Here's how the part is built. I have some questions about the finished solid (model axes, mm). Round coordinates to 2 decimals unless told otherwise and drop trailing zeros. Write each loop counter-clockwise with the first axis right and the second up, starting at its lowest first coordinate (ties: lowest second). Pieces come first, ordered by that corner, then holes. Notation, with made-up numbers: (66.25, 63) -> (117.25, 63) arc R26 cw to (117.25, 93) -> close; hole circle Ø10 at (74, -21). An arc over 180 degrees is marked (long way). Put each result on its own line as item: value. Start each with the question number.
1) If I drill on line 1 along Y through (x, z) = (30, 0.35); line 2 along Y through (x, z) = (50, 2); line 3 along Y through (x, z) = (-10, 0.05), over which ranges is the centre line in solid material (lowest first)? Write a range as [from, to].
2) I want a section at D-D, the plane x = 50. List the corners of the cut face in (y, z) for me.
3) I want a section at B-B, the plane x = 90. List the corners of the cut face in (y, z) for me, then the cut area to 3 significant figures.
4) Will this pin go through, and if not, where does the flat tip stop? P1, Ø5.5, axis at x = 90, y = -52.5, coming from the -Z side.
5) I want a section at A-A, the plane z = 0. List the corners of the cut face in (x, y) for me, then the cut area to 3 significant figures.
6) I want a section at C-C, the plane y = -52.5. List the corners of the cut face in (x, z) for me, then the cut area to 3 significant figures.
from build123d import *

# Parameters (mm, degrees)
SKETCH_1_R          = 5
EXTRUDE_1_DEPTH     = 3
SKETCH_2_R          = 2.1
CUT_EXTRUDE_1_DEPTH = 119.077305186
CHAMFER_1_SIZE      = 30
CHAMFER_3_SIZE      = 4
CHAMFER_2_SIZE      = 2


with BuildPart() as part:
    # 草图1 → 凸台-拉伸1 (new, symmetric)
    with BuildSketch(Plane.XY):
        Polygon((-20, 52.5), (-20, -62.5), (100, -62.5), (100, -42.5), (60, 52.5), align=None)
        Circle(SKETCH_1_R, mode=Mode.SUBTRACT)
    extrude(amount=EXTRUDE_1_DEPTH, both=True)

    # 草图2 → 切除-拉伸1 (cut, through all)
    with BuildSketch(Plane.XY.offset(3)):
        with Locations((-10, 42.5)):
            Circle(SKETCH_2_R)
        with Locations((30, 42.5)):
            Circle(SKETCH_2_R)
        with Locations((50, 42.5)):
            Circle(SKETCH_2_R)
        with Locations((50, -32.5)):
            Circle(SKETCH_2_R)
        with Locations((30, -52.5)):
            Circle(SKETCH_2_R)
        with Locations((90, -52.5)):
            Circle(SKETCH_2_R)
    extrude(amount=-CUT_EXTRUDE_1_DEPTH, mode=Mode.SUBTRACT)

    # 倒角1
    chamfer_1_edges = [part.edges().sort_by_distance(p)[0] for p in [
        (-20, -62.5, 0),
    ]]
    chamfer(chamfer_1_edges, length=CHAMFER_1_SIZE)

    # 倒角3
    chamfer_3_edges = [part.edges().sort_by_distance(p)[0] for p in [
        (100, -62.5, 0),
        (-20, 52.5, 0),
    ]]
    chamfer(chamfer_3_edges, length=CHAMFER_3_SIZE)

    # 倒角2
    chamfer_2_edges = [part.edges().sort_by_distance(p)[0] for p in [
        (47.9, 42.5, -3),
        (47.9, -32.5, -3),
        (27.9, -52.5, -3),
        (87.9, -52.5, -3),
    ]]
    chamfer(chamfer_2_edges, length=CHAMFER_2_SIZE)


solid = part.part
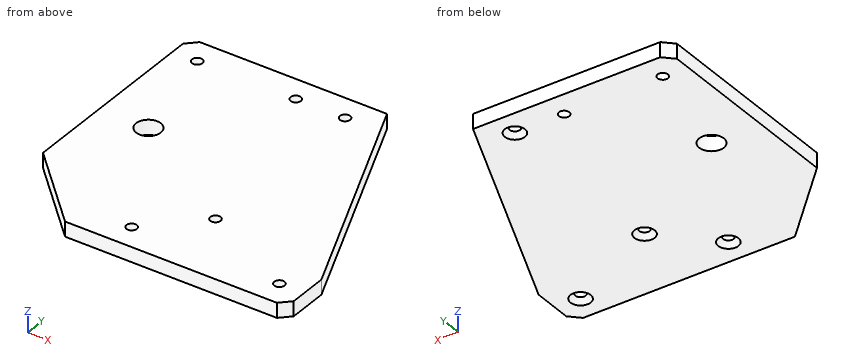
Findings:
1. line 1: y = [-62.5, -54.6], [-50.4, 40.4], [44.6, 52.5]
1. line 2: y = [-62.5, -34.6], [-30.4, 40.4], [44.6, 52.5]
1. line 3: y = [-42.5, 40.4], [44.6, 52.5]
2. outline: (-62.5, -3) -> (-36.6, -3) -> (-34.6, -1) -> (-34.6, 3) -> (-62.5, 3) -> close; (-30.4, -1) -> (-28.4, -3) -> (38.4, -3) -> (40.4, -1) -> (40.4, 3) -> (-30.4, 3) -> close; (44.6, -1) -> (46.6, -3) -> (52.5, -3) -> (52.5, 3) -> (44.6, 3) -> close
3. outline: (-62.5, -3) -> (-56.6, -3) -> (-54.6, -1) -> (-54.6, 3) -> (-62.5, 3) -> close; (-50.4, -1) -> (-48.4, -3) -> (-18.75, -3) -> (-18.75, 3) -> (-50.4, 3) -> close
3. area: 233 mm2
4. P1: stops at z = -1.65
5. outline: (-20, -32.5) -> (10, -62.5) -> (96, -62.5) -> (100, -58.5) -> (100, -42.5) -> (60, 52.5) -> (-16, 52.5) -> (-20, 48.5) -> close; hole circle Ø4.2 at (-10, 42.5); hole circle Ø10 at (0, 0); hole circle Ø4.2 at (30, -52.5); hole circle Ø4.2 at (30, 42.5); hole circle Ø4.2 at (50, -32.5); hole circle Ø4.2 at (50, 42.5); hole circle Ø4.2 at (90, -52.5)
5. area: 11,300 mm2
6. outline: (0, -3) -> (25.9, -3) -> (27.9, -1) -> (27.9, 3) -> (0, 3) -> close; (32.1, -1) -> (34.1, -3) -> (85.9, -3) -> (87.9, -1) -> (87.9, 3) -> (32.1, 3) -> close; (92.1, -1) -> (94.1, -3) -> (100, -3) -> (100, 3) -> (92.1, 3) -> close
6. area: 542 mm2
